The model under review builds one solid part; all positions refer to its coordinate system, in mm. Face numbers are marked on the shaded views. A direction names the side the tool comes from. Round coordinates to 2 decimals unless told otherwise and drop trailing zeros. Loops run counter-clockwise (first coordinate to the right, second up) from the corner with the lowest first, then second, coordinate; pieces in that order, holes last. Notation, with made-up numbers: (-5, -4) -> (19, -4) arc R21 ccw to (19, 1) -> close; hole circle Ø3 at (5.25, 0). An arc over 180 degrees is marked (long way). Write each question's results on one line, items separated by ' | '. Start each with the question number.
Item 1: For L1, parallel to Y at x = 0, z = -9.1; L2, parallel to X at y = 3.1, z = 17.5, list the stretches that pass through material, from the lowest coordinate up. Write a range as from..to.
Item 2: We need section D-D (y = 8.25). Give the boundary of the cut face in (x, z), and give its area (3 significant figures).
Item 3: Tool access review of the marked faces 5 and 6: name each direction out of +Z, -Z, +X, -X, +Y, -Y from which nothing blocks a thin tool from reaching the whole face with its end or side.
Item 4: We need section B-B (z = 0). Give the boundary of the cut face in (x, y), and give its area (3 significant figures).
Item 5: Mouldability with a two-part tool opening along Y and no side actions: class the marked faces 1, 2, 3 and 4 as pulls with the +Y half, pulls with the -Y half, needs draft (parallel to the pull), parting line crosses it, or undercut.
Item 6: We need section C-C (x = 17.5). Give the boundary of the cut face in (y, z), and give its area (4 significant figures).
Item 7: Clearance check with flat-ended pins moving along their axes: pin 1 Ø6.5 at (y, z) = (12, -2) entering from +X; pin 2 Ø10.5 at (x, y) = (2.5, 15) entering from +Z; pin 3 Ø12 at (x, y) = (6, 12.5) entering from -Z; pin 4 Ø1.1 at (x, y) = (-8, 12) entering from +Z. State where each tip first meets the part, or that it passes through.
Item 8: We need section A-A (y = 12.5). Give the boundary of the cut face in (x, z).
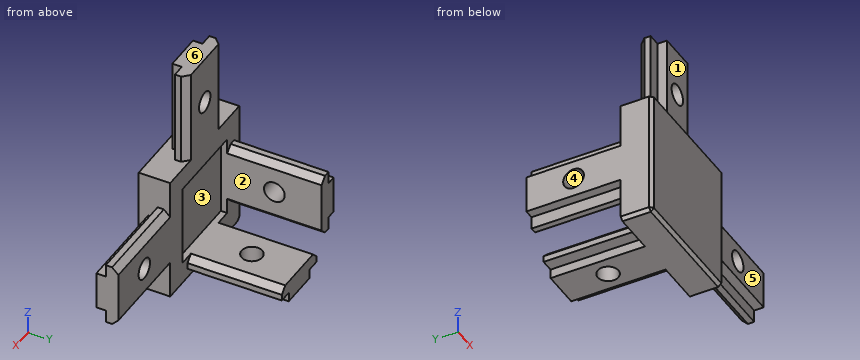
from build123d import *

# Parameters (mm, degrees)
SKETCH_1_W          = 20
SKETCH_1_H          = 20
EXTRUDE_1_DEPTH     = 5
EXTRUDE_3_DEPTH     = 15
EXTRUDE_4_DEPTH     = 15
EXTRUDE_5_DEPTH     = 15
SKETCH_9_W          = 13
SKETCH_9_H          = 13
CUT_EXTRUDE_4_DEPTH = 1
HOLE_WIZARD_M4_1_D  = 3.3
HOLE_WIZARD_M4_2_D  = 3.3
HOLE_WIZARD_M4_3_D  = 3.3
CHAMFER_1_SIZE      = 0.5


with BuildPart() as part:
    # 草图1 → 凸台-拉伸1 (new body)
    with BuildSketch(Plane(origin=(0, 0, 0), x_dir=(1, 0, 0), z_dir=(0, 1, 0))):
        Rectangle(SKETCH_1_W, SKETCH_1_H)
    extrude(amount=EXTRUDE_1_DEPTH)

    # 草图6 → 凸台-拉伸3 (add)
    with BuildSketch(Plane(origin=(10, 0, 0), x_dir=(0, 0, -1), z_dir=(1, 0, 0))):
        Polygon((-3, 1.5), (-3, 3), (-5, 3), (-5, 4), (-4, 5), (4, 5), (5, 4), (5, 3), (3, 3), (3, 1.5), align=None)
    extrude(amount=EXTRUDE_3_DEPTH)

    # 草图7 → 凸台-拉伸4 (add)
    with BuildSketch(Plane.XY.offset(10)):
        Polygon((-3, 1.5), (-3, 3), (-5, 3), (-5, 4), (-4, 5), (4, 5), (5, 4), (5, 3), (3, 3), (3, 1.5), align=None)
    extrude(amount=EXTRUDE_4_DEPTH)

    # 草图8 → 凸台-拉伸5 (add)
    with BuildSketch(Plane(origin=(0, 5, 0), x_dir=(1, 0, 0), z_dir=(0, 1, 0))):
        Polygon((-10, 3), (-8.5, 3), (-8.5, 5), (-7.5, 5), (-6.5, 4), (-6.5, -4), (-7.5, -5), (-8.5, -5), (-8.5, -3), (-10, -3), align=None)
        Polygon((3, 10), (-3, 10), (-3, 8.5), (-5, 8.5), (-5, 7.5), (-4, 6.5), (4, 6.5), (5, 7.5), (5, 8.5), (3, 8.5), align=None)
    extrude(amount=EXTRUDE_5_DEPTH)

    # 草图9 → 切除-拉伸4 (cut)
    with BuildSketch(Plane(origin=(0, 5, 0), x_dir=(1, 0, 0), z_dir=(0, 1, 0))):
        Rectangle(SKETCH_9_W, SKETCH_9_H)
    extrude(amount=-CUT_EXTRUDE_4_DEPTH, mode=Mode.SUBTRACT)

    # M4 螺纹孔1 (through all)
    with Locations(Plane(origin=(0, 5, 0), x_dir=(1, 0, 0), z_dir=(0, 1, 0))):
        with Locations((0, -17.5), (17.5, 0)):
            Hole(HOLE_WIZARD_M4_1_D / 2)

    # M4 螺纹孔2 (through all)
    with Locations(Plane.XY.offset(-6.5)):
        with Locations((0, 12.5)):
            Hole(HOLE_WIZARD_M4_2_D / 2)

    # M4 螺纹孔3 (through all)
    with Locations(Plane(origin=(-6.5, 0, 0), x_dir=(0, 0, -1), z_dir=(1, 0, 0))):
        with Locations((0, 12.5)):
            Hole(HOLE_WIZARD_M4_3_D / 2)

    # 倒角1
    chamfer_1_edges = [part.edges().sort_by_distance(p)[0] for p in [
        (-10, 0, 0),
        (0, 0, -10),
        (-10, 2.5, -10),
    ]]
    chamfer(chamfer_1_edges, length=CHAMFER_1_SIZE)


solid = part.part
Here are the results:
1) L1: y = 0..10.85, 14.15..20 | L2: x = -5..-1.65, 1.65..5
2) outline: (-10, -3) -> (-8.5, -3) -> (-8.5, -5) -> (-7.5, -5) -> (-6.5, -4) -> (-6.5, 4) -> (-7.5, 5) -> (-8.5, 5) -> (-8.5, 3) -> (-10, 3) -> close; (-5, -8.5) -> (-3, -8.5) -> (-3, -10) -> (3, -10) -> (3, -8.5) -> (5, -8.5) -> (5, -7.5) -> (4, -6.5) -> (-4, -6.5) -> (-5, -7.5) -> close | area: 56.0 mm2
3) face 5: +Z, -Z, +X, -Y | face 6: +Z, +X, -X, +Y, -Y
4) outline: (-10, 0.5) -> (-9.5, 0) -> (10, 0) -> (10, 1.5) -> (15.85, 1.5) -> (15.85, 5) -> (6.5, 5) -> (6.5, 4) -> (-6.5, 4) -> (-6.5, 10.85) -> (-10, 10.85) -> close; (-10, 14.15) -> (-6.5, 14.15) -> (-6.5, 20) -> (-10, 20) -> close; (19.15, 1.5) -> (25, 1.5) -> (25, 5) -> (19.15, 5) -> close | area: 169 mm2
5) face 1: pulls with the -Y half | face 2: needs draft | face 3: pulls with the +Y half | face 4: undercut
6) outline: (1.5, -3) -> (3, -3) -> (3, -5) -> (4, -5) -> (5, -4) -> (5, -1.65) -> (1.5, -1.65) -> close; (1.5, 1.65) -> (5, 1.65) -> (5, 4) -> (4, 5) -> (3, 5) -> (3, 3) -> (1.5, 3) -> close | area: 16.45 mm2
7) pin 1: stops at x = -6.5 | pin 2: stops at z = -6.5 | pin 3: stops at z = -10 | pin 4: stops at z = 5
8) outline: (-10, -3) -> (-8.5, -3) -> (-8.5, -5) -> (-7.5, -5) -> (-6.5, -4) -> (-6.5, -1.65) -> (-10, -1.65) -> close; (-10, 1.65) -> (-6.5, 1.65) -> (-6.5, 4) -> (-7.5, 5) -> (-8.5, 5) -> (-8.5, 3) -> (-10, 3) -> close; (-5, -8.5) -> (-3, -8.5) -> (-3, -10) -> (-1.65, -10) -> (-1.65, -6.5) -> (-4, -6.5) -> (-5, -7.5) -> close; (1.65, -10) -> (3, -10) -> (3, -8.5) -> (5, -8.5) -> (5, -7.5) -> (4, -6.5) -> (1.65, -6.5) -> close
